Check sheet for the drawn part. Datum: minimum x, y, z corner. Units: mm. Give positions to 0.01 mm unless a question says otherwise; leave off trailing zeros. Loops run counter-clockwise (first coordinate to the right, second up) from the corner with the lowest first, then second, coordinate; pieces in that order, holes last. Notation, with made-up numbers: M 47.25,6 L 70.25,6 A17 ccw 70.25,32 Z; hole C -18,-37.5 d3. An arc over 180 degrees is marked long. Write each question's results on one line, items separated by ' | '. Start each with the question number.
1. Sectioned sample at B-B on z = 3.75. Record the cut outline in (x, y).
2. Sectioned sample at C-C on y = 9.75. Record the cut outline in (x, z), and give its area (3 significant figures).
3. Go/stop test with flat-tipped pins: pin 1 (7.5 mm diameter, centred on x = 62.26, y = 7, fed in from -Z); pin 2 (1.5 mm diameter, centred on y = 6, z = 1.5, fed in from +X); pin 3 (1.5 mm diameter, centred on y = 3, z = 3, fed in from +X); pin 4 (3 mm diameter, centred on y = 4, z = 3, fed in from -X). Record where each tip stops, or that it passes through.
4. Sectioned sample at A-A on y = 5.5. Record the cut outline in (x, z), and give its area (3 significant figures).
5. Material ranges on line 1 along X through (y, z) = (5.25, 1.1); line 2 along Y through (x, z) = (62.26, 2.15); line 3 along X through (y, z) = (4.25, 3.75), recorded low to high.
6. Draft check along X on the marked faces 1 and 2. Enter one of: pulls with the +X half, pulls with the -X half, needs draft (parallel to the pull), parting line crosses it, or undercut.
7. Sectioned sample at D-D on y = 1. Record the cut outline in (x, z).
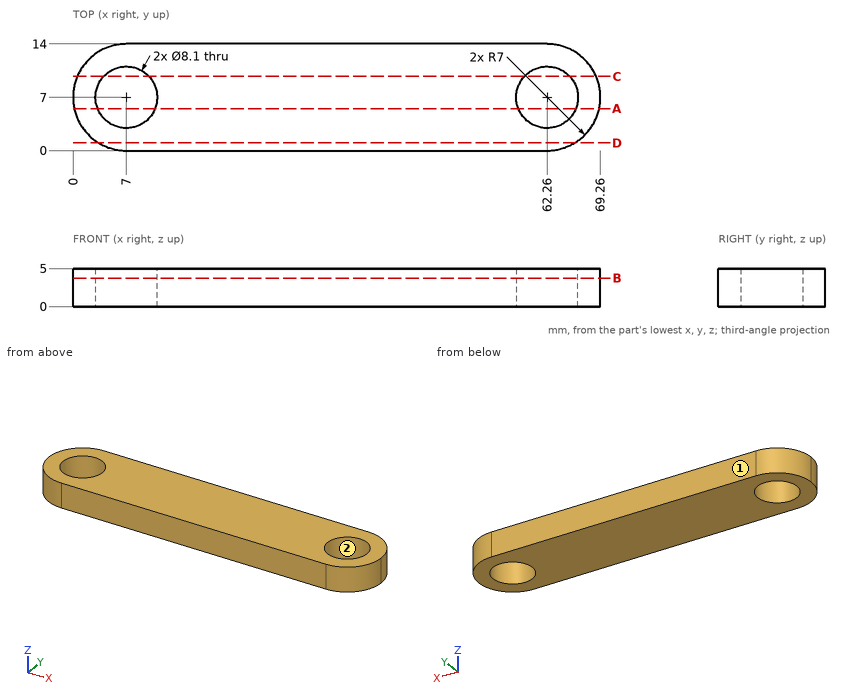
Output values:
1) outline: M 7,0 L 62.26,0 A7 ccw 62.26,14 L 7,14 A7 ccw Z; hole C 7,7 d8.1; hole C 62.26,7 d8.1
2) outline: M 0.56,0 L 4.03,0 L 4.03,5 L 0.56,5 Z; M 9.97,0 L 59.29,0 L 59.29,5 L 9.97,5 Z; M 65.23,0 L 68.7,0 L 68.7,5 L 65.23,5 Z | area: 281 mm2
3) pin 1: through | pin 2: x = 69.26 | pin 3: x = 68.46 | pin 4: x = 0.16
4) outline: M 0.16,0 L 3.24,0 L 3.24,5 L 0.16,5 Z; M 10.76,0 L 58.5,0 L 58.5,5 L 10.76,5 Z; M 66.02,0 L 69.1,0 L 69.1,5 L 66.02,5 Z | area: 269 mm2
5) line 1: 0.22 to 3.35, 10.65 to 58.61, 65.91 to 69.04 | line 2: 0 to 2.95, 11.05 to 14 | line 3: 0.56 to 4.03, 9.97 to 59.29, 65.23 to 68.7
6) face 1: needs draft | face 2: undercut
7) outline: M 3.39,0 L 65.87,0 L 65.87,5 L 3.39,5 Z
